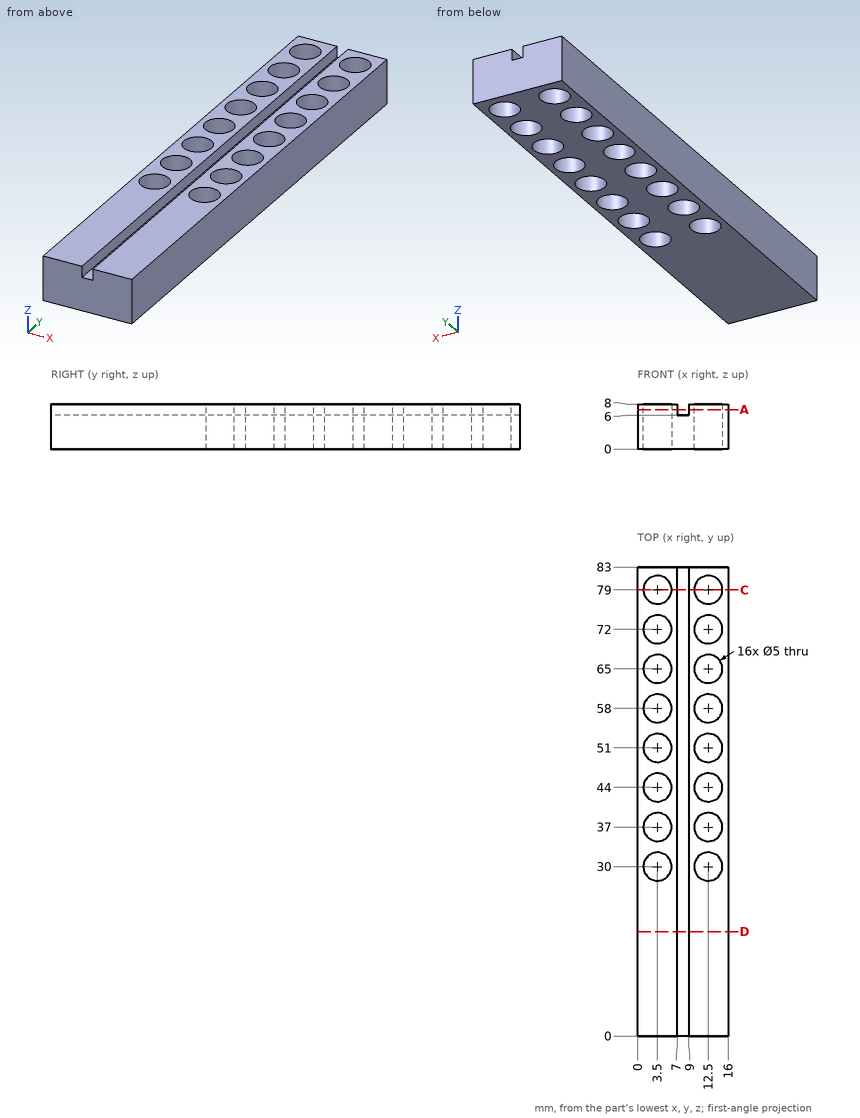
Input: dimensioned drawing with shaded views. Units: mm. Origin: part minimum x, y, z. Coordinates: 2 decimals unless noted, no trailing zeros. Order: outer loops, then holes, each group sorted by start corner. A loop starts at its lowest first (then second) coordinate and runs counter-clockwise, first axis right, second up. Notation, with made-up numbers: (40, 70) - (61, 70) arc R11 cw to (61, 84) - close; hole circle Ø11 at (45.5, 14.25). An arc over 180 degrees is marked (long way). Put each result on its own line as item: value.
1. Contact query for flat-ended pins moving along their axis: pin 1 Ø3 at (x, y) = (3.5, 37) entering from -Z; pin 2 Ø0.6 at (x, y) = (8, 27) entering from +Z. Output: stop coordinate, or through.
Report:
pin 1: passes through
pin 2: stops at z = 6
2. Line query: line 1 along X through (y, z) = (63, 4.5); line 2 along X through (y, z) = (59, 6.75); line 3 along X through (y, z) = (73.5, 5.75). Output: solid intervals per line, ascending.
Report:
line 1: x = 0 to 2, 5 to 11, 14 to 16
line 2: x = 0 to 1.21, 5.79 to 7, 9 to 10.21, 14.79 to 16
line 3: x = 0 to 1.5, 5.5 to 10.5, 14.5 to 16
3. Cut plane C-C on y = 79. Return the cut outline in (x, z).
Report:
outline: (0, 0) - (1, 0) - (1, 8) - (0, 8) - close; (6, 0) - (10, 0) - (10, 8) - (9, 8) - (9, 6) - (7, 6) - (7, 8) - (6, 8) - close; (15, 0) - (16, 0) - (16, 8) - (15, 8) - close
4. Cut plane A-A on z = 7. State how many separate pieces and enclosed holes the cut face has, then the cut area to 3 significant figures.
Report:
separate pieces: 2
enclosed holes: 16
area: 848 mm2
5. Cut plane D-D on y = 18.5. Return the cut outline in (x, z).
Report:
outline: (0, 0) - (16, 0) - (16, 8) - (9, 8) - (9, 6) - (7, 6) - (7, 8) - (0, 8) - close
